Design review of the part built by this model. Coordinates are the model's own, in mm. A direction names the side the tool comes from. Coordinates: 2 decimals unless noted, no trailing zeros. Return JSON: item names as keys, results as strings. Group by question number.
```python
from build123d import *

# Parameters (mm, degrees)
SKETCH1_W           = 21.411233639
SKETCH1_H           = 96.993593864
BOSS_EXTRUDE1_DEPTH = 3


with BuildPart() as part:
    # Sketch1 → Boss-Extrude1 (new body)
    with BuildSketch(Plane.XY):
        with Locations((-91.64577638, 82.405352126)):
            Rectangle(SKETCH1_W, SKETCH1_H)
        with BuildLine():
            Line((-86.19596438, 38.053580074), (-95.937669189, 38.053580074))
            ThreePointArc((-95.937669189, 38.053580074), (-97.965327886, 40.081238771), (-95.937669189, 42.108897468))
            Line((-95.937669189, 42.108897468), (-86.19596438, 42.108897468))
            ThreePointArc((-86.19596438, 42.108897468), (-84.168305683, 40.081238771), (-86.19596438, 38.053580074))
        make_face(mode=Mode.SUBTRACT)
        with BuildLine():
            Line((-86.19596438, 48.053580074), (-95.937669189, 48.053580074))
            ThreePointArc((-95.937669189, 48.053580074), (-97.965327886, 50.081238771), (-95.937669189, 52.108897468))
            Line((-95.937669189, 52.108897468), (-86.19596438, 52.108897468))
            ThreePointArc((-86.19596438, 52.108897468), (-84.168305683, 50.081238771), (-86.19596438, 48.053580074))
        make_face(mode=Mode.SUBTRACT)
        with BuildLine():
            Line((-86.19596438, 58.053580074), (-95.937669189, 58.053580074))
            ThreePointArc((-95.937669189, 58.053580074), (-97.965327886, 60.081238771), (-95.937669189, 62.108897468))
            Line((-95.937669189, 62.108897468), (-86.19596438, 62.108897468))
            ThreePointArc((-86.19596438, 62.108897468), (-84.168305683, 60.081238771), (-86.19596438, 58.053580074))
        make_face(mode=Mode.SUBTRACT)
        with BuildLine():
            Line((-86.19596438, 68.053580074), (-95.937669189, 68.053580074))
            ThreePointArc((-95.937669189, 68.053580074), (-97.965327886, 70.081238771), (-95.937669189, 72.108897468))
            Line((-95.937669189, 72.108897468), (-86.19596438, 72.108897468))
            ThreePointArc((-86.19596438, 72.108897468), (-84.168305683, 70.081238771), (-86.19596438, 68.053580074))
        make_face(mode=Mode.SUBTRACT)
        with BuildLine():
            Line((-86.19596438, 78.053580074), (-95.937669189, 78.053580074))
            ThreePointArc((-95.937669189, 78.053580074), (-97.965327886, 80.081238771), (-95.937669189, 82.108897468))
            Line((-95.937669189, 82.108897468), (-86.19596438, 82.108897468))
            ThreePointArc((-86.19596438, 82.108897468), (-84.168305683, 80.081238771), (-86.19596438, 78.053580074))
        make_face(mode=Mode.SUBTRACT)
        with BuildLine():
            Line((-86.19596438, 88.053580074), (-95.937669189, 88.053580074))
            ThreePointArc((-95.937669189, 88.053580074), (-97.965327886, 90.081238771), (-95.937669189, 92.108897468))
            Line((-95.937669189, 92.108897468), (-86.19596438, 92.108897468))
            ThreePointArc((-86.19596438, 92.108897468), (-84.168305683, 90.081238771), (-86.19596438, 88.053580074))
        make_face(mode=Mode.SUBTRACT)
        with BuildLine():
            Line((-86.19596438, 98.053580074), (-95.937669189, 98.053580074))
            ThreePointArc((-95.937669189, 98.053580074), (-97.965327886, 100.081238771), (-95.937669189, 102.108897468))
            Line((-95.937669189, 102.108897468), (-86.19596438, 102.108897468))
            ThreePointArc((-86.19596438, 102.108897468), (-84.168305683, 100.081238771), (-86.19596438, 98.053580074))
        make_face(mode=Mode.SUBTRACT)
        with BuildLine():
            Line((-86.19596438, 108.053580074), (-95.937669189, 108.053580074))
            ThreePointArc((-95.937669189, 108.053580074), (-97.965327886, 110.081238771), (-95.937669189, 112.108897468))
            Line((-95.937669189, 112.108897468), (-86.19596438, 112.108897468))
            ThreePointArc((-86.19596438, 112.108897468), (-84.168305683, 110.081238771), (-86.19596438, 108.053580074))
        make_face(mode=Mode.SUBTRACT)
        with BuildLine():
            Line((-86.19596438, 118.053580074), (-95.937669189, 118.053580074))
            ThreePointArc((-95.937669189, 118.053580074), (-97.965327886, 120.081238771), (-95.937669189, 122.108897468))
            Line((-95.937669189, 122.108897468), (-86.19596438, 122.108897468))
            ThreePointArc((-86.19596438, 122.108897468), (-84.168305683, 120.081238771), (-86.19596438, 118.053580074))
        make_face(mode=Mode.SUBTRACT)
    extrude(amount=BOSS_EXTRUDE1_DEPTH)


solid = part.part
```
Item 1: Machinability: for faces 1 (the flat face through (-91, 62.109, 1)), 2 (the flat face through (-80.94, 82, 1)), which of the approach directions +Z, -Z, +X, -X, +Y, -Y give a long, thin tool a straight path to every point of the face, cutting with its end or side? Answer none if there is none.
Item 2: The part is to be moulded in two halves that separate along Y. For faces 3 (the flat face through (-91, 38.054, 1)), 4 (the flat face through (-102.351, 82, 1)), say which applies: pulls with the +Y half, pulls with the -Y half, needs draft (parallel to the pull), parting line crosses it, or undercut.
Item 3: Add section A-A (z = 1.9). Count the separate pieces of the cut face and the enclosed holes in it, plus the area to 3 significant figures.
Item 4: For line 1 (X direction, y = 69, z = 1.4); line 2 (X direction, y = 78.5, z = 1.2), list the stretches that pass through material, from the lowest coordinate up.
Geometry check:
{
 "1": {"face 1": "+Z, -Z", "face 2": "+Z, -Z, +X, +Y, -Y"},
 "2": {"face 3": "undercut", "face 4": "needs draft"},
 "3": {"separate pieces": "1", "enclosed holes": "9", "area": "1,600 mm^2"},
 "4": {"line 1": "-102.35 to -97.65, -84.48 to -80.94", "line 2": "-102.35 to -97.21, -84.93 to -80.94"}
}
